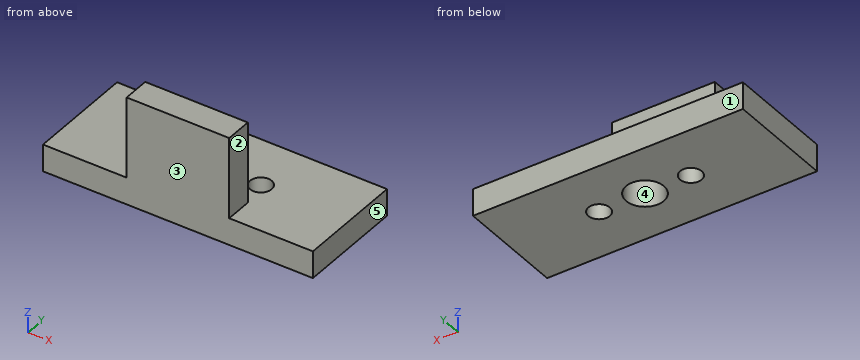
Autodesk Inventor part; units mm, degrees
ref_plane "YZ Plane" through (0, 0, 0) normal (1, 0, 0) x (0, 1, 0)
ref_plane "XZ Plane" through (0, 0, 0) normal (0, 1, 0) x (-1, 0, 0)
ref_plane "XY Plane" through (0, 0, 0) normal (0, 0, 1) x (1, 0, 0)
sketch "Sketch1" plane through (0, 0, 0) normal (0, 0, 1) x (1, 0, 0)
  line L0 (0, 0) -> (50, 0)
  circle A0 centre (25, 10) radius 3.5
  line L1 (0, 0) -> (0, 20)
  line L2 (0, 20) -> (50, 20)
  line L3 (50, 20) -> (50, 0)
  point P0 (25, 0)
  dimension "d0" = 50
  dimension "d2" = 7
  dimension "d3" = 10
  dimension "d4" = 20
extrude "Extrusion1" add sketch "Sketch1" along normal blind 5
sketch "Sketch2" plane through (0, 0, 5) normal (0, 0, 1) x (1, 0, 0)
  line L0 (0, 0) -> (50, 0)
  line L1 (15.5, 0) -> (34.5, 0)
  line L2 (34.5, 0) -> (34.5, 5)
  line L3 (34.5, 5) -> (15.5, 5)
  line L4 (15.5, 5) -> (15.5, 0)
  point P0 (25, 0)
  dimension "d7" = 19
  dimension "d8" = 5
extrude "Extrusion2" add sketch "Sketch2" along normal blind 15
sketch "Sketch3" plane through (0, 0, 5) normal (0, 0, 1) x (1, 0, 0)
  circle A0 centre (16.5, 10) radius 2
  circle A1 centre (33.5, 10) radius 2
  line L0 (34.5, 5) -> (34.5, 0)
  line L1 (34.5, 0) -> (50, 0)
  line L2 (50, 0) -> (50, 20)
  line L3 (50, 20) -> (0, 20)
  line L4 (0, 20) -> (0, 0)
  line L5 (0, 0) -> (15.5, 0)
  line L6 (15.5, 0) -> (15.5, 5)
  line L7 (15.5, 5) -> (34.5, 5)
  circle A2 centre (25, 10) radius 3.5
  line L8 (16.5, 10) -> (33.5, 10) construction
  dimension "d11" = 4
  dimension "d12" = 4
  dimension "d13" = 17
extrude "Extrusion3" cut sketch "Sketch3" against normal through all contours A0 | A1
properties part number "C005" material "Steel, Carbon"
Source: CAD feature listing. Evaluate the final solid. Frame: model axes, mm. Face numbers are marked on the shaded views. A direction names the side the tool comes from. Coordinates: 2 decimals unless noted, no trailing zeros. Loops run counter-clockwise (first coordinate to the right, second up) from the corner with the lowest first, then second, coordinate; pieces in that order, holes last. Notation, with made-up numbers: (35.5, 78.25) -> (63.5, 78.25) arc R13 ccw to (63.5, 94.25) -> close; hole circle Ø9 at (28.5, -16). An arc over 180 degrees is marked (long way). Answer in a Markdown table with one row per item. Add a question column.
Q1. Contact query for flat-ended pins moving along their axis: pin 1 Ø1.5 at (y, z) = (17, 6) entering from +X; pin 2 Ø5.5 at (y, z) = (3, 14.5) entering from -X; pin 3 Ø5.5 at (y, z) = (2, 9) entering from +X; pin 4 Ø12 at (x, z) = (20.5, 14.5) entering from +Y. Output: stop coordinate, or through.
Q2. Pull-direction query (Y, two-part tool) for the marked faces 3, 4 and 5; classes: pulls with the +Y half, pulls with the -Y half, needs draft (parallel to the pull), parting line crosses it, or undercut.
Q3. Ray query, line 1 along Y through (x, z) = (16.5, 2.2); line 2 along X through (y, z) = (9.25, 2.75); line 3 along Z through (x, y) = (10.5, 16.5). Return the intervals inside material, ascending.
Q4. Section C-C on y = 7. Return the cut outline in (x, z), and give its area (3 significant figures).
Q5. Reachability of the marked faces 1 and 2 from +Z, -Z, +X, -X, +Y, -Y: full face, straight path, thin tool, end or side. Return the list, or none.
Q6. Section A-A on x = 16.5. Return the cut outline in (y, z), and give its area (3 significant figures).
Q7. Section D-D on x = 25. Return the cut outline in (y, z).
Q8. Section B-B on y = 10. Return the cut outline in (x, z), and give its area (3 significant figures).
Computed values:
| question | item | result |
|---|---|---|
| 1 | pin 1 | passes through |
| 1 | pin 2 | stops at x = 15.5 |
| 1 | pin 3 | stops at x = 34.5 |
| 1 | pin 4 | stops at y = 5 |
| 2 | face 3 | pulls with the -Y half |
| 2 | face 4 | undercut |
| 2 | face 5 | needs draft |
| 3 | line 1 | y = 0 to 8, 12 to 20 |
| 3 | line 2 | x = 0 to 14.65, 18.35 to 21.58, 28.42 to 31.65, 35.35 to 50 |
| 3 | line 3 | z = 0 to 5 |
| 4 | outline | (0, 0) -> (23.2, 0) -> (23.2, 5) -> (0, 5) -> close; (26.8, 0) -> (50, 0) -> (50, 5) -> (26.8, 5) -> close |
| 4 | area | 232 mm^2 |
| 5 | face 1 | +Z, -Z, +X, -X, +Y |
| 5 | face 2 | +Z, +X, +Y, -Y |
| 6 | outline | (0, 0) -> (8, 0) -> (8, 5) -> (5, 5) -> (5, 20) -> (0, 20) -> close; (12, 0) -> (20, 0) -> (20, 5) -> (12, 5) -> close |
| 6 | area | 155 mm^2 |
| 7 | outline | (0, 0) -> (6.5, 0) -> (6.5, 5) -> (5, 5) -> (5, 20) -> (0, 20) -> close; (13.5, 0) -> (20, 0) -> (20, 5) -> (13.5, 5) -> close |
| 8 | outline | (0, 0) -> (14.5, 0) -> (14.5, 5) -> (0, 5) -> close; (18.5, 0) -> (21.5, 0) -> (21.5, 5) -> (18.5, 5) -> close; (28.5, 0) -> (31.5, 0) -> (31.5, 5) -> (28.5, 5) -> close; (35.5, 0) -> (50, 0) -> (50, 5) -> (35.5, 5) -> close |
| 8 | area | 175 mm^2 |
